The listing builds one solid part. Answer for the finished solid, in the listing's coordinates (mm). A direction names the side the tool comes from. Give positions to 0.01 mm unless a question says otherwise; leave off trailing zeros. Loops run counter-clockwise (first coordinate to the right, second up) from the corner with the lowest first, then second, coordinate; pieces in that order, holes last. Notation, with made-up numbers: (62, 14) - (110, 14) arc R27 ccw to (110, 33) - close; hole circle Ø5 at (19, 1). An arc over 180 degrees is marked (long way). Answer as CSV lines item,"result". Start each with the question number.
1) A cutting plane is placed at A-A (y = 6.75). Give the number of separate pieces and of enclosed holes in the cut face, and give its area (3 significant figures).
2) Find the intervals of material crossed by line 1 along Z through (x, y) = (-2.5, 4.5); line 2 along X through (y, z) = (3.5, -6); line 3 along X through (y, z) = (1.5, 17.5), in increasing order.
3) Flat-ended cylindrical pins translate along their axes: pin 1 (1.5 mm diameter, centred on x = -7.5, y = 4.5, fed in from +Z); pin 2 (1.6 mm diameter, centred on x = 0.5, z = 24.5, fed in from -Y); pin 3 (2 mm diameter, centred on y = 6.5, z = 19, fed in from +X); pin 4 (4 mm diameter, centred on y = 2.5, z = 15, fed in from -X). Find the tip coordinate at first contact, or state that the pin passes through.
4) A cutting plane is placed at B-B (z = 9.5). Determine the outline of the cut face in (x, y), and give its area (3 significant figures).
5) For faces 1 (the face through (2.262, 2.465, 26.282)), 2 (the face through (-5.837, 3.944, 2.854)), determine the directions among +Z, -Z, +X, -X, +Y, -Y from which every point of the face is accessible in a straight line to the end or side of a thin tool.
6) For a pull along X with two mould halves and no side action, classify faces 3 (the face through (0, 4, -10)), 4 (the face through (6.4, 3.94, -0.42)), 5 (the face through (6.38, 3.94, 0.55)) as pulls with the +X half, pulls with the -X half, needs draft (parallel to the pull), parting line crosses it, or undercut.
```python
from build123d import *

# Parameters (mm, degrees)
SKETCH1_R           = 10
SKETCH1_R_2         = 5.6
BOSS_EXTRUDE1_DEPTH = 8
CUT_EXTRUDE1_START  = -8
CUT_EXTRUDE1_DEPTH  = 8
BOSS_EXTRUDE2_START = -8
SKETCH3_R           = 2
BOSS_EXTRUDE2_DEPTH = 8
CUT_EXTRUDE2_DEPTH  = 5


with BuildPart() as part:
    # Sketch1 → Boss-Extrude1 (new body)
    with BuildSketch(Plane(origin=(0, 0, 0), x_dir=(1, 0, 0), z_dir=(0, 1, 0))):
        with Locations(Location((0, 0, 0), (0, 0, 270))):
            Circle(SKETCH1_R)
        with Locations(Location((0, 0, 0), (0, 0, 270))):
            Circle(SKETCH1_R_2, mode=Mode.SUBTRACT)
    extrude(amount=BOSS_EXTRUDE1_DEPTH)

    # Sketch2 → Cut-Extrude1 (cut)
    with BuildSketch(Plane(origin=(0, 8, 0), x_dir=(1, 0, 0), z_dir=(0, 1, 0)).offset(CUT_EXTRUDE1_START)):
        with BuildLine():
            ThreePointArc((0.064249913, 6.948346368), (0, 6.971717727), (-0.064249913, 6.948346368))
            ThreePointArc((-0.064249913, 6.948346368), (-0.498286109, 6.437987083), (-0.739423422, 5.812921636))
            ThreePointArc((-0.739423422, 5.812921636), (-0.850059891, 5.608071058), (-1.056027259, 5.499527837))
            ThreePointArc((-1.056027259, 5.499527837), (0, 5.6), (1.056027259, 5.499527837))
            ThreePointArc((1.056027259, 5.499527837), (0.850059891, 5.608071058), (0.739423422, 5.812921636))
            ThreePointArc((0.739423422, 5.812921636), (0.498286109, 6.437987083), (0.064249913, 6.948346368))
        make_face()
        with BuildLine():
            ThreePointArc((-3.07784083, 4.678343278), (-2.13595945, 5.176647296), (-1.116741665, 5.487521121))
            ThreePointArc((-1.116741665, 5.487521121), (-1.350243109, 5.510209511), (-1.530862217, 5.659923992))
            ThreePointArc((-1.530862217, 5.659923992), (-1.996402784, 6.157420979), (-2.601935295, 6.469769583))
            ThreePointArc((-2.601935295, 6.469769583), (-2.670238307, 6.466774526), (-2.720653655, 6.420594828))
            ThreePointArc((-2.720653655, 6.420594828), (-2.927784399, 5.772859186), (-2.905902141, 5.093163831))
            ThreePointArc((-2.905902141, 5.093163831), (-2.928170827, 4.859350312), (-3.07784083, 4.678343278))
        make_face()
        with BuildLine():
            ThreePointArc((1.546699763, 5.647927275), (1.366304802, 5.503873184), (1.136351309, 5.483493932))
            ThreePointArc((1.136351309, 5.483493932), (2.145111804, 5.172861428), (3.077665403, 4.678458685))
            ThreePointArc((3.077665403, 4.678458685), (2.929649667, 4.855512924), (2.904074445, 5.084865862))
            ThreePointArc((2.904074445, 5.084865862), (2.914679464, 5.743680773), (2.710627264, 6.370188757))
            ThreePointArc((2.710627264, 6.370188757), (2.660211916, 6.416368455), (2.591908904, 6.419363512))
            ThreePointArc((2.591908904, 6.419363512), (2.004925243, 6.120871804), (1.546699763, 5.647927275))
        make_face()
        with BuildLine():
            ThreePointArc((-4.626747894, 3.154869874), (-3.942798212, 3.976725067), (-3.115113277, 4.653608199))
            ThreePointArc((-3.115113277, 4.653608199), (-3.341080574, 4.586023742), (-3.565845172, 4.65750628))
            ThreePointArc((-3.565845172, 4.65750628), (-4.193243775, 4.947890892), (-4.882025833, 5.007317379))
            ThreePointArc((-4.882025833, 5.007317379), (-4.943983429, 4.978411876), (-4.972888932, 4.916454281))
            ThreePointArc((-4.972888932, 4.916454281), (-4.914521213, 4.231672555), (-4.62778579, 3.607080208))
            ThreePointArc((-4.62778579, 3.607080208), (-4.55723094, 3.381135785), (-4.626747894, 3.154869874))
        make_face()
        with BuildLine():
            ThreePointArc((3.60147946, 4.613515157), (3.380624437, 4.551916923), (3.162225119, 4.621723953))
            ThreePointArc((3.162225119, 4.621723953), (3.969775698, 3.949795047), (4.637621263, 3.138864289))
            ThreePointArc((4.637621263, 3.138864289), (4.568924656, 3.357086949), (4.631064299, 3.577266461))
            ThreePointArc((4.631064299, 3.577266461), (4.885266795, 4.17532686), (4.934309795, 4.823316006))
            ThreePointArc((4.934309795, 4.823316006), (4.905404292, 4.885273602), (4.843446696, 4.914179105))
            ThreePointArc((4.843446696, 4.914179105), (4.197804444, 4.865705756), (3.60147946, 4.613515157))
        make_face()
        with BuildLine():
            ThreePointArc((-5.477673311, 1.164085519), (-5.155741489, 2.185939087), (-4.645101504, 3.127783883))
            ThreePointArc((-4.645101504, 3.127783883), (-4.829188719, 2.979467261), (-5.064867635, 2.960991018))
            ThreePointArc((-5.064867635, 2.960991018), (-5.762609895, 2.993266281), (-6.428898584, 2.783634848))
            ThreePointArc((-6.428898584, 2.783634848), (-6.475078282, 2.7332195), (-6.478073339, 2.664916489))
            ThreePointArc((-6.478073339, 2.664916489), (-6.160056055, 2.051923175), (-5.652515264, 1.58363038))
            ThreePointArc((-5.652515264, 1.58363038), (-5.499714793, 1.401104329), (-5.477673311, 1.164085519))
        make_face()
        with BuildLine():
            ThreePointArc((5.102964873, 2.86242986), (4.876497297, 2.891701995), (4.702948527, 3.040111043))
            ThreePointArc((4.702948527, 3.040111043), (5.186580684, 2.111724605), (5.488979978, 1.109548918))
            ThreePointArc((5.488979978, 1.109548918), (5.509040687, 1.335802715), (5.649058612, 1.51465515))
            ThreePointArc((5.649058612, 1.51465515), (6.106834087, 1.967933206), (6.396761999, 2.543225468))
            ThreePointArc((6.396761999, 2.543225468), (6.393766942, 2.61152848), (6.347587244, 2.661943828))
            ThreePointArc((6.347587244, 2.661943828), (5.741485734, 2.862816923), (5.102964873, 2.86242986))
        make_face()
        with BuildLine():
            ThreePointArc((-5.510664325, -0.996282441), (-5.599538908, 0.071861119), (-5.483282283, 1.137372148))
            ThreePointArc((-5.483282283, 1.137372148), (-5.597366262, 0.930602816), (-5.808201648, 0.824220718))
            ThreePointArc((-5.808201648, 0.824220718), (-6.468837551, 0.587557408), (-7.007056195, 0.137257497))
            ThreePointArc((-7.007056195, 0.137257497), (-7.030427554, 0.073007584), (-7.007056195, 0.008757671))
            ThreePointArc((-7.007056195, 0.008757671), (-6.479586979, -0.435338259), (-5.8326499, -0.673911904))
            ThreePointArc((-5.8326499, -0.673911904), (-5.621271562, -0.784771791), (-5.510664325, -0.996282441))
        make_face()
        with BuildLine():
            ThreePointArc((5.812810952, 0.664521681), (5.615514351, 0.779198979), (5.513031953, 0.983096477))
            ThreePointArc((5.513031953, 0.983096477), (5.599695706, -0.058378103), (5.49133793, -1.097819539))
            ThreePointArc((5.49133793, -1.097819539), (5.59652681, -0.897662861), (5.793441288, -0.786522929))
            ThreePointArc((5.793441288, -0.786522929), (6.388422373, -0.542837618), (6.875338784, -0.122959741))
            ThreePointArc((6.875338784, -0.122959741), (6.898710143, -0.058709827), (6.875338784, 0.005540086))
            ThreePointArc((6.875338784, 0.005540086), (6.396892952, 0.420193633), (5.812810952, 0.664521681))
        make_face()
        with BuildLine():
            ThreePointArc((-4.723716983, -3.00773966), (-5.209771972, -2.053844201), (-5.505416772, -1.024883487))
            ThreePointArc((-5.505416772, -1.024883487), (-5.532233953, -1.25849938), (-5.685687223, -1.436678055))
            ThreePointArc((-5.685687223, -1.436678055), (-6.204243765, -1.907832783), (-6.52847941, -2.528927711))
            ThreePointArc((-6.52847941, -2.528927711), (-6.525484353, -2.597230723), (-6.479304655, -2.647646071))
            ThreePointArc((-6.479304655, -2.647646071), (-5.827313187, -2.855366074), (-5.14346104, -2.83114388))
            ThreePointArc((-5.14346104, -2.83114388), (-4.906005926, -2.853880543), (-4.723716983, -3.00773966))
        make_face()
        with BuildLine():
            ThreePointArc((-3.231573409, -4.573503395), (-4.040870944, -3.877030051), (-4.703269727, -3.0396141))
            ThreePointArc((-4.703269727, -3.0396141), (-4.639287647, -3.264216822), (-4.711631901, -3.486267262))
            ThreePointArc((-4.711631901, -3.486267262), (-5.005567924, -4.11636587), (-5.066027207, -4.809018249))
            ThreePointArc((-5.066027207, -4.809018249), (-5.037121704, -4.870975845), (-4.975164108, -4.899881348))
            ThreePointArc((-4.975164108, -4.899881348), (-4.301827611, -4.844494009), (-3.685350478, -4.568078128))
            ThreePointArc((-3.685350478, -4.568078128), (-3.457618103, -4.500210794), (-3.231573409, -4.573503395))
        make_face()
        with BuildLine():
            ThreePointArc((5.618520803, -1.63637781), (5.480067966, -1.454143469), (5.464186765, -1.225831555))
            ThreePointArc((5.464186765, -1.225831555), (5.14101235, -2.220358534), (4.638570438, -3.13746144))
            ThreePointArc((4.638570438, -3.13746144), (4.812780485, -2.993714728), (5.037083425, -2.967248735))
            ThreePointArc((5.037083425, -2.967248735), (5.683333022, -2.971442449), (6.297181173, -2.769337092))
            ThreePointArc((6.297181173, -2.769337092), (6.343360871, -2.718921743), (6.346355928, -2.650618732))
            ThreePointArc((6.346355928, -2.650618732), (6.063599568, -2.085255724), (5.618520803, -1.63637781))
        make_face()
        with BuildLine():
            ThreePointArc((-1.251247201, -5.45842289), (-2.260605052, -5.123442671), (-3.188432984, -4.603682777))
            ThreePointArc((-3.188432984, -4.603682777), (-3.044381817, -4.784979292), (-3.024926972, -5.015718698))
            ThreePointArc((-3.024926972, -5.015718698), (-3.05036452, -5.701707725), (-2.842344676, -6.355891))
            ThreePointArc((-2.842344676, -6.355891), (-2.791929328, -6.402070698), (-2.723626316, -6.405065755))
            ThreePointArc((-2.723626316, -6.405065755), (-2.131541606, -6.102796604), (-1.671238282, -5.623159457))
            ThreePointArc((-1.671238282, -5.623159457), (-1.48668328, -5.475931261), (-1.251247201, -5.45842289))
        make_face()
        with BuildLine():
            ThreePointArc((4.553131765, -3.68047341), (4.494207557, -3.457914037), (4.567722636, -3.239739175))
            ThreePointArc((4.567722636, -3.239739175), (3.883669423, -4.034490279), (3.063445285, -4.68778231))
            ThreePointArc((3.063445285, -4.68778231), (3.280286024, -4.622628788), (3.497760134, -4.685635919))
            ThreePointArc((3.497760134, -4.685635919), (4.09857718, -4.943062107), (4.750308422, -4.993019623))
            ThreePointArc((4.750308422, -4.993019623), (4.812266018, -4.964114119), (4.841171521, -4.902156524))
            ThreePointArc((4.841171521, -4.902156524), (4.795474246, -4.268133163), (4.553131765, -3.68047341))
        make_face()
        with BuildLine():
            ThreePointArc((0.925303441, -5.52302576), (-0.130378711, -5.598482061), (-1.181403822, -5.473964286))
            ThreePointArc((-1.181403822, -5.473964286), (-0.980381907, -5.584707692), (-0.873319684, -5.787714078))
            ThreePointArc((-0.873319684, -5.787714078), (-0.632839966, -6.418904201), (-0.195967325, -6.934048611))
            ThreePointArc((-0.195967325, -6.934048611), (-0.131717411, -6.95741997), (-0.067467498, -6.934048611))
            ThreePointArc((-0.067467498, -6.934048611), (0.357915774, -6.438102524), (0.600752826, -5.831518965))
            ThreePointArc((0.600752826, -5.831518965), (0.715816891, -5.627603722), (0.925303441, -5.52302576))
        make_face()
        with BuildLine():
            ThreePointArc((2.787896701, -5.152413925), (2.8176875, -4.922252146), (2.970261988, -4.747372297))
            ThreePointArc((2.970261988, -4.747372297), (2.028927178, -5.219526272), (1.015839733, -5.507092666))
            ThreePointArc((1.015839733, -5.507092666), (1.242257752, -5.531230611), (1.418818304, -5.675015626))
            ThreePointArc((1.418818304, -5.675015626), (1.878837632, -6.153725835), (2.470217884, -6.455471826))
            ThreePointArc((2.470217884, -6.455471826), (2.538520896, -6.452476769), (2.588936244, -6.406297071))
            ThreePointArc((2.588936244, -6.406297071), (2.790550207, -5.795561613), (2.787896701, -5.152413925))
        make_face()
    extrude(amount=CUT_EXTRUDE1_DEPTH, mode=Mode.SUBTRACT)

    # Sketch3 → Boss-Extrude2 (add)
    with BuildSketch(Plane(origin=(0, 8, 0), x_dir=(1, 0, 0), z_dir=(0, 1, 0)).offset(BOSS_EXTRUDE2_START)):
        with BuildLine():
            Line((-5, -8.660254038), (-5, -21.68337521))
            ThreePointArc((-5, -21.68337521), (0, -31), (5, -21.68337521))
            Line((5, -21.68337521), (5, -8.660254038))
            ThreePointArc((5, -8.660254038), (0, -10), (-5, -8.660254038))
        make_face()
        with Locations(Location((0, -25, 0), (0, 0, 270))):
            Circle(SKETCH3_R, mode=Mode.SUBTRACT)
    extrude(amount=BOSS_EXTRUDE2_DEPTH)

    # Sketch4 → Cut-Extrude2 (cut)
    with BuildSketch(Plane.XZ):
        Polygon((1.5011107, 27.6), (-1.5011107, 27.6), (-3.0022214, 25), (-1.5011107, 22.4), (1.5011107, 22.4), (3.0022214, 25), align=None)
    extrude(amount=-CUT_EXTRUDE2_DEPTH, mode=Mode.SUBTRACT)


solid = part.part
```
Ans:
1,separate pieces,"1"
1,enclosed holes,"2"
1,area,"395 mm2"
2,line 1,"-9.68 to -6.43, 6.32 to 24.13, 25.87 to 30.45"
2,line 2,"-8 to -2.88, -1.81 to -0.69, 0.69 to 1.86, 2.86 to 8"
2,line 3,"-5 to 5"
3,pin 1,"z = 7.38"
3,pin 2,"through"
3,pin 3,"x = 5"
3,pin 4,"x = -5"
4,outline,"(-5, 0) - (5, 0) - (5, 8) - (-5, 8) - close"
4,area,"80.0 mm2"
5,face 1,"-Y"
5,face 2,"+Y, -Y"
6,face 3,"parting line crosses it"
6,face 4,"undercut"
6,face 5,"undercut"
